from build123d import *

# Parameters (mm, degrees)
SKETCH_1_W          = 12
SKETCH_1_H          = 12
SKETCH_1_W_2        = 9
SKETCH_1_H_2        = 9
EXTRUDE_1_DEPTH     = 241
SKETCH_2_R          = 1.6
CUT_EXTRUDE_1_DEPTH = 13
SKETCH_3_R          = 1.6
CUT_EXTRUDE_2_DEPTH = 13
SKETCH_4_R          = 1.6
CUT_EXTRUDE_3_DEPTH = 13


with BuildPart() as part:
    # ｽｹｯﾁ1 → ﾎﾞｽ - 押し出し1 (new body)
    with BuildSketch(Plane(origin=(0, 0, 0), x_dir=(0, 0, -1), z_dir=(1, 0, 0))):
        with Locations((6, 6)):
            Rectangle(SKETCH_1_W, SKETCH_1_H)
        with Locations((6, 6)):
            Rectangle(SKETCH_1_W_2, SKETCH_1_H_2, mode=Mode.SUBTRACT)
    extrude(amount=EXTRUDE_1_DEPTH)

    # ｽｹｯﾁ2 → ｶｯﾄ - 押し出し1 (cut, through all)
    with BuildSketch(Plane(origin=(0, 12, 0), x_dir=(1, 0, 0), z_dir=(0, 1, 0))):
        with Locations((18, 6)):
            Circle(SKETCH_2_R)
        with Locations((223, 6)):
            Circle(SKETCH_2_R)
    extrude(amount=-CUT_EXTRUDE_1_DEPTH, mode=Mode.SUBTRACT)

    # ｽｹｯﾁ3 → ｶｯﾄ - 押し出し2 (cut, through all)
    with BuildSketch(Plane.XY):
        with Locations((6, 6)):
            Circle(SKETCH_3_R)
        with Locations((235, 6)):
            Circle(SKETCH_3_R)
    extrude(amount=-CUT_EXTRUDE_2_DEPTH, mode=Mode.SUBTRACT)

    # ｽｹｯﾁ4 → ｶｯﾄ - 押し出し3 (cut, through all)
    with BuildSketch(Plane.XZ):
        with Locations((42, -6)):
            Circle(SKETCH_4_R)
        with Locations((72, -6)):
            Circle(SKETCH_4_R)
        with Locations((169, -6)):
            Circle(SKETCH_4_R)
        with Locations((199, -6)):
            Circle(SKETCH_4_R)
    extrude(amount=-CUT_EXTRUDE_3_DEPTH, mode=Mode.SUBTRACT)


solid = part.part
Geometry check sheet. Reference: the model listing, model coordinates, mm. A direction names the side the tool comes from. Give positions to 0.01 mm unless a question says otherwise; leave off trailing zeros. Loops run counter-clockwise (first coordinate to the right, second up) from the corner with the lowest first, then second, coordinate; pieces in that order, holes last. Notation, with made-up numbers: (57, 29.25) -> (103, 29.25) arc R14 cw to (103, 52.25) -> close; hole circle Ø10 at (6, 4). An arc over 180 degrees is marked (long way). Answer in a Markdown table with one row per item. Add a question column.
1) Material ranges on probe 1 along Y at (x, z) = (105, -2.25); probe 2 along Z at (x, y) = (126, 4); probe 3 along Z at (x, y) = (42, 1.15), recorded low to high. Write a range as from..to.
2) Gauge pin test, flat end, axial feed: P1, Ø3, axis at x = 235, y = 6, coming from the -Z side. Record the tip position at first contact, or that the pin passes through.
3) Cross-section at A-A on x = 102. Record the boundary of the cut face in (y, z), and give its area (3 significant figures).
4) Set-up check for faces 1 (the face through (241, 6, -11)), 2 (the face through (119, 6, -1.5)): record each of +Z, -Z, +X, -X, +Y, -Y from which the full face is reachable in a straight line by a thin tool's end or side.
Outcome:
| question | item | result |
|---|---|---|
| 1 | probe 1 | y = 0..1.5, 10.5..12 |
| 1 | probe 2 | z = -12..-10.5, -1.5..0 |
| 1 | probe 3 | z = -12..-7.6, -4.4..0 |
| 2 | P1 | passes through |
| 3 | outline | (0, -12) -> (12, -12) -> (12, 0) -> (0, 0) -> close; hole (1.5, -10.5) -> (10.5, -10.5) -> (10.5, -1.5) -> (1.5, -1.5) -> close |
| 3 | area | 63.0 mm^2 |
| 4 | face 1 | +Z, -Z, +X, +Y, -Y |
| 4 | face 2 | +X, -X |
